from build123d import *

# Parameters (mm, degrees)
SKETCH1_R           = 2
BOSS_EXTRUDE1_DEPTH = 3


with BuildPart() as part:
    # Sketch1 → Boss-Extrude1 (new body)
    with BuildSketch(Plane(origin=(0, 0, 0), x_dir=(0, 0, -1), z_dir=(1, 0, 0))):
        Polygon((0, 0), (25, 35), (45, 35), (70, 0), (70, -23), (0, -23), align=None)
        with Locations((35, -13)):
            Circle(SKETCH1_R, mode=Mode.SUBTRACT)
        with Locations((35, 29)):
            Circle(SKETCH1_R, mode=Mode.SUBTRACT)
    extrude(amount=BOSS_EXTRUDE1_DEPTH)


solid = part.part
For this review, take the finished solid that the model builds, in its own axes (mm). Round coordinates to 2 decimals unless told otherwise and drop trailing zeros. Write each loop counter-clockwise with the first axis right and the second up, starting at its lowest first coordinate (ties: lowest second). Pieces come first, ordered by that corner, then holes. Notation, with made-up numbers: (17, 85.25) -> (68, 85.25) arc R22 ccw to (68, 107.25) -> close; hole circle Ø6 at (-6, 3.25). An arc over 180 degrees is marked (long way). Put each result on its own line as item: value.
Q1. The part is to be moulded in two halves that separate along Y. For faces 1 (the flat face through (3, 0, -35)), 2 (the flat face through (1, 35, -35)), 3 (the cylindrical face through (1.479, 27.226, -35.923)), say which applies: released by +Y, released by -Y, zero draft, split by the parting line, or undercut.
Determined:
face 1: zero draft
face 2: released by +Y
face 3: undercut
Q2. Consider section A-A on y = -13. State the section outline as (x, z) points.
Determined:
outline: (0, -70) -> (3, -70) -> (3, -37) -> (0, -37) -> close; (0, -33) -> (3, -33) -> (3, 0) -> (0, 0) -> close
Q3. Consider section D-D on y = 29. State the section outline as (x, z) points, and give its area (3 significant figures).
Determined:
outline: (0, -49.29) -> (3, -49.29) -> (3, -37) -> (0, -37) -> close; (0, -33) -> (3, -33) -> (3, -20.71) -> (0, -20.71) -> close
area: 73.7 mm^2
Q4. Consider section C-C on z = -35. State the section outline as (x, y) points.
Determined:
outline: (0, -23) -> (3, -23) -> (3, -15) -> (0, -15) -> close; (0, -11) -> (3, -11) -> (3, 27) -> (0, 27) -> close; (0, 31) -> (3, 31) -> (3, 35) -> (0, 35) -> close
Q5. To check wall thickness, follow L1, parallel to Y at x = 1.4, z = -35; L2, parallel to Z at x = 1.5, y = 21; L3, parallel to Z at x = 2.45, y = 30. State the ranges of each line that lie inside material, in increasing order. Write a range as [from, to].
Determined:
L1: y = [-23, -15], [-11, 27], [31, 35]
L2: z = [-55, -15]
L3: z = [-48.57, -36.73], [-33.27, -21.43]
Q6. Consider section B-B on x = 1.5. State the section outline as (y, z) points.
Determined:
outline: (-23, -70) -> (0, -70) -> (35, -45) -> (35, -25) -> (0, 0) -> (-23, 0) -> close; hole circle Ø4 at (-13, -35); hole circle Ø4 at (29, -35)
